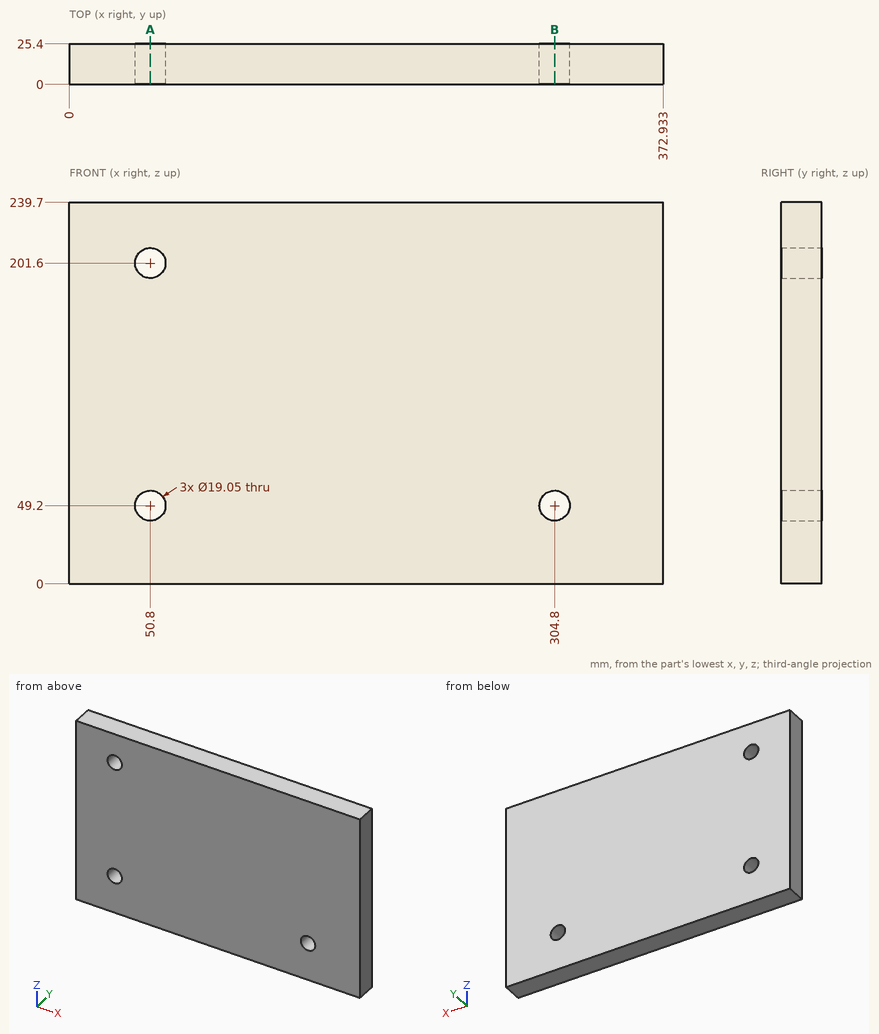
Answer from the drawing. Dimensions are ordinates in mm from the lowest x, y and z of the part. Coordinates: 2 decimals unless noted, no trailing zeros. Loops run counter-clockwise (first coordinate to the right, second up) from the corner with the lowest first, then second, coordinate; pieces in that order, holes last.
Q1. This flat-tipped pin is pushed along its axis until it touches: pin 1 Ø17 at (x, z) = (50.8, 49.2) entering from +Y. Where does it stop, or does it pass through?
Q2. The part is cut by section B-B on x = 304.8. Write down the section's boundary in (y, z) (1 decimal), and give its area (3 significant figures).
Q3. The part is cut by section A-A on x = 50.8. Write down the section's boundary in (y, z) (1 decimal).
Q4. Consider probe 1 along Z at (x, y) = (304.8, 13.75) (1 decimal); probe 2 along Z at (x, y) = (58.5, 12.25) (1 decimal); probe 3 along Z at (x, y) = (51, 4.5). Determine where each line is inside the solid, lowest interval first.
Results below:
1. pin 1: passes through
2. outline: (0, 0) - (25.4, 0) - (25.4, 39.7) - (0, 39.7) - close; (0, 58.7) - (25.4, 58.7) - (25.4, 239.7) - (0, 239.7) - close
2. area: 5,600 mm2
3. outline: (0, 0) - (25.4, 0) - (25.4, 39.7) - (0, 39.7) - close; (0, 58.7) - (25.4, 58.7) - (25.4, 192.1) - (0, 192.1) - close; (0, 211.1) - (25.4, 211.1) - (25.4, 239.7) - (0, 239.7) - close
4. probe 1: z = 0 to 39.7, 58.7 to 239.7
4. probe 2: z = 0 to 43.6, 54.8 to 196, 207.2 to 239.7
4. probe 3: z = 0 to 39.68, 58.72 to 192.08, 211.12 to 239.7
